from build123d import *

# Parameters (mm, degrees)
BOSS_EXTRUDE1_DEPTH = 1219.2
FILLET1_R           = 0.381
FILLET2_R           = 1.5875


with BuildPart() as part:
    # Sketch2 → Boss-Extrude1 (new body)
    with BuildSketch(Plane.XY):
        Polygon((0, 0), (0, 50.8), (9.525, 50.8), (9.525, 41.275), (2.032, 41.275), (2.032, 25.4), (3.0734, 9.525), (57.15, 9.525), (57.15, 0), (47.625, 0), (47.625, 7.493), (28.575, 7.493), (9.525, 6.4516), (9.525, 0), align=None)
    extrude(amount=BOSS_EXTRUDE1_DEPTH)

    # Fillet1
    fillet1_edges = [part.edges().sort_by_distance(p)[0] for p in [
        (0, 0, 609.6),
        (0, 50.8, 609.6),
        (9.525, 50.8, 609.6),
        (9.525, 41.275, 609.6),
        (2.032, 41.275, 609.6),
        (57.15, 9.525, 609.6),
        (57.15, 0, 609.6),
        (47.625, 0, 609.6),
        (47.625, 7.493, 609.6),
        (9.525, 0, 609.6),
    ]]
    fillet(fillet1_edges, radius=FILLET1_R)

    # Fillet2
    fillet2_edges = [part.edges().sort_by_distance(p)[0] for p in [
        (3.0734, 9.525, 609.6),
        (9.525, 6.4516, 609.6),
    ]]
    fillet(fillet2_edges, radius=FILLET2_R)


solid = part.part
Model file for the job. Use its own axes, mm. Give positions to 0.01 mm unless a question says otherwise; leave off trailing zeros. Use one line per item in the form item = value.
(1) Drop flat-ended pins along their axis: P1, Ø12.5, axis at y = 31.5, z = 504.5, coming from the +X side; P2, Ø2.5, axis at y = 46.5, z = 772.5, coming from the +X side (3 decimals); P3, Ø20.5, axis at x = 34, z = 525, coming from the -Y side. Give the stop position or say it passes through.
Determined:
P1 = 2.04
P2 = 9.525
P3 = 7.23
(2) Pull direction X, two halves, no side cores. Call faces 1 (the face through (0, 25, 601)), 2 (the face through (20, 9, 0)), 3 (the face through (38, 7.493, 601)): pulls with the +X half, pulls with the -X half, needs draft (parallel to the pull), parting line crosses it, or undercut.
Determined:
face_1 = pulls with the -X half
face_2 = needs draft
face_3 = undercut
(3) Drill centre lines: L1, parallel to Y at x = 8.5, z = 592 (3 decimals); L2, parallel to Y at x = 13.5, z = 394.5 (3 decimals); L3, parallel to Y at x = 27.5, z = 675.5 (3 decimals). Where is each one in solid material? Low to high.
Determined:
L1 = 0 to 9.525, 41.275 to 50.8
L2 = 6.669 to 9.525
L3 = 7.434 to 9.525
